from build123d import *

# Parameters (mm, degrees)
EXTRUDE_1_DEPTH     = 8
CUT_EXTRUDE_1_REACH = 53.614
SKETCH_2_R          = 3
CUT_EXTRUDE_START   = -3
CUT_EXTRUDE_2_DEPTH = 3
CUT_EXTRUDE_3_REACH = 53.614
SKETCH_4_R          = 1.7
CUT_EXTRUDE_4_REACH = 53.614
FILLET_2_R          = 2


# Read off the part's stored shape, not the designer's step: the extrude step
with BuildPart() as part:
    # Sketch 1 → Extrude 1 (new body)
    with BuildSketch(Plane(origin=(0, 0, 0), x_dir=(1, 0, 0), z_dir=(0, 1, 0))):
        with BuildLine():
            Line((5, 8.660254038), (5, 45))
            ThreePointArc((5, 45), (0, 50), (-5, 45))
            Line((-5, 45), (-5, 8.660254038))
            ThreePointArc((-5, 8.660254038), (0, -10), (5, 8.660254038))
        make_face()
    extrude(amount=EXTRUDE_1_DEPTH)

    # Sketch 2 → Cut-Extrude 1 (cut, up to next)
    with BuildSketch(Plane(origin=(0, 8, 0), x_dir=(1, 0, 0), z_dir=(0, 1, 0)), mode=Mode.PRIVATE) as cut_extrude_1_sk1:
        with Locations(Location((0, 0, 0), (0, 0, 270))):
            Circle(SKETCH_2_R)
    cut_extrude_1_tool1 = extrude(cut_extrude_1_sk1.sketch, amount=-CUT_EXTRUDE_1_REACH, mode=Mode.PRIVATE) & part.part
    add(cut_extrude_1_tool1.solids().sort_by_distance((0, 8, 0))[0], mode=Mode.SUBTRACT)

    # Cut-Extrude 2 outline → Cut-Extrude 2 (cut)
    with BuildSketch(Plane.XZ.offset(CUT_EXTRUDE_START)):
        with BuildLine():
            Line((1.898730713, -10.628348376), (2.982064694, -0.327551768))
            ThreePointArc((2.982064694, -0.327551768), (-0.01385186, -2.999968021), (-2.984962311, -0.3))
            Line((-2.984962311, -0.3), (-1.989974874, -10.2))
            ThreePointArc((-1.989974874, -10.2), (-0.218979353, -11.987975866), (1.898730713, -10.628348376))
        make_face()
    extrude(amount=CUT_EXTRUDE_2_DEPTH, mode=Mode.SUBTRACT)

    # Sketch 4 → Cut-Extrude 3 (cut, up to next)
    with BuildSketch(Plane(origin=(0, 8, 0), x_dir=(1, 0, 0), z_dir=(0, 1, 0)), mode=Mode.PRIVATE) as cut_extrude_3_sk1:
        with Locations(Location((0, 45, 0), (0, 0, 270))):
            Circle(SKETCH_4_R)
    cut_extrude_3_tool1 = extrude(cut_extrude_3_sk1.sketch, amount=-CUT_EXTRUDE_3_REACH, mode=Mode.PRIVATE) & part.part
    add(cut_extrude_3_tool1.solids().sort_by_distance((0, 8, -45))[0], mode=Mode.SUBTRACT)

    # Sketch 5 → Cut-Extrude 4 (cut, up to next)
    with BuildSketch(Plane.XZ, mode=Mode.PRIVATE) as cut_extrude_4_sk1:
        with BuildLine():
            Line((-2.5, -36.830127019), (-2.5, -16.830127019))
            ThreePointArc((-2.5, -16.830127019), (0, -14.330127019), (2.5, -16.830127019))
            Line((2.5, -16.830127019), (2.5, -36.830127019))
            ThreePointArc((2.5, -36.830127019), (0, -39.330127019), (-2.5, -36.830127019))
        make_face()
    cut_extrude_4_tool1 = extrude(cut_extrude_4_sk1.sketch, amount=-CUT_EXTRUDE_4_REACH, mode=Mode.PRIVATE) & part.part
    add(cut_extrude_4_tool1.solids().sort_by_distance((0, 0, -26.830127))[0], mode=Mode.SUBTRACT)

    # Fillet 2
    fillet_2_edges = [part.edges().sort_by_distance(p)[0] for p in [
        (0, 8, -50),
        (-5, 8, -26.830127019),
        (0, 8, 10),
        (5, 8, -26.830127019),
        (0, 0, 10),
        (-5, 0, -26.830127019),
        (0, 0, -50),
        (5, 0, -26.830127019),
    ]]
    fillet(fillet_2_edges, radius=FILLET_2_R)


solid = part.part
CAD build for the part. Positions are in the model's coordinates, mm. A direction names the side the tool comes from. Coordinates: 2 decimals unless noted, no trailing zeros. Loops run counter-clockwise (first coordinate to the right, second up) from the corner with the lowest first, then second, coordinate; pieces in that order, holes last. Notation, with made-up numbers: (82.5, -27.75) - (124.5, -27.75) arc R16 ccw to (124.5, -10.75) - close; hole circle Ø5 at (-18, 12). An arc over 180 degrees is marked (long way). Use one line per item in the form item = value. Start each with the question number.
1) Tool access for faces 4 (the face through (-0.05, 3.94, -14.33)), 5 (the face through (0, 3, -7)), 6 (the face through (4.4, 0.57, -26.47)), 7 (the face through (5, 4, -27)), 8 (the face through (-4.43, 7.4, -25.95)): list every direction of +Z, -Z, +X, -X, +Y, -Y with a clear straight run to the whole face (end or side of a thin tool).
2) Band-saw the part on B-B (z = -33.5). Give the cut face in (x, y), and give its area (3 significant figures).
3) Flat gauge pins, fed straight in: pin 1 (1.5 mm diameter, centred on y = 3.5, z = -27, fed in from -X); pin 2 (2 mm diameter, centred on y = 5, z = -27, fed in from +X); pin 3 (3 mm diameter, centred on x = 0, z = -45, fed in from -Y); pin 4 (1 mm diameter, centred on y = 1, z = -14.5, fed in from +X). Where does each tip first touch, or does it go through?
4) Band-saw the part on C-C (z = -41). Give the cut face in (x, y), and give its area (3 significant figures).
5) Two-plate mould, pull along X, no slides. Class faces 1 (the face through (1, 0, -12)), 2 (the face through (-5, 4, -27)), 3 (the face through (0.9, 4.94, 2.86)): +X half, -X half, draft (parallel to the pull), parting line (faces both ways), or undercut.
6) Band-saw the part on A-A (x = 0). Give the cut face in (y, z).
7) Drill centre lines: L1, parallel to X at y = 5.5, z = 0; L2, parallel to X at y = 3, z = -45; L3, parallel to Y at x = 0, z = -8. Where is each one in solid material? Low to high. Write a range as from..to.
Check values:
q1.face_4 = +Y, -Y
q1.face_5 = -Y
q1.face_6 = -Z, +X, -Y
q1.face_7 = -Z, +X, +Y, -Y
q1.face_8 = -Z, -X, +Y
q2.outline = (-5, 2) arc R2 ccw to (-3, 0) - (-2.5, 0) - (-2.5, 8) - (-3, 8) arc R2 ccw to (-5, 6) - close; (2.5, 0) - (3, 0) arc R2 ccw to (5, 2) - (5, 6) arc R2 ccw to (3, 8) - (2.5, 8) - close
q2.area = 36.6 mm2
q3.pin_1 = -5
q3.pin_2 = 5
q3.pin_3 = through
q3.pin_4 = 4.94
q4.outline = (-5, 2) arc R2 ccw to (-3, 0) - (3, 0) arc R2 ccw to (5, 2) - (5, 6) arc R2 ccw to (3, 8) - (-3, 8) arc R2 ccw to (-5, 6) - close
q4.area = 76.6 mm2
q5.face_1 = draft
q5.face_2 = -X half
q5.face_3 = undercut
q6.outline = (0, -48) arc R2 ccw to (2, -50) - (6, -50) arc R2 ccw to (8, -48) - (8, -46.7) - (0, -46.7) - close; (0, -43.3) - (8, -43.3) - (8, -39.33) - (0, -39.33) - close; (0, -14.33) - (8, -14.33) - (8, -3) - (3, -3) - (3, -12) - (0, -12) - close; (0, 3) - (8, 3) - (8, 8) arc R2 ccw to (6, 10) - (2, 10) arc R2 ccw to (0, 8) - close
q7.L1 = -10..-3, 3..10
q7.L2 = -5..-1.7, 1.7..5
q7.L3 = 3..8
